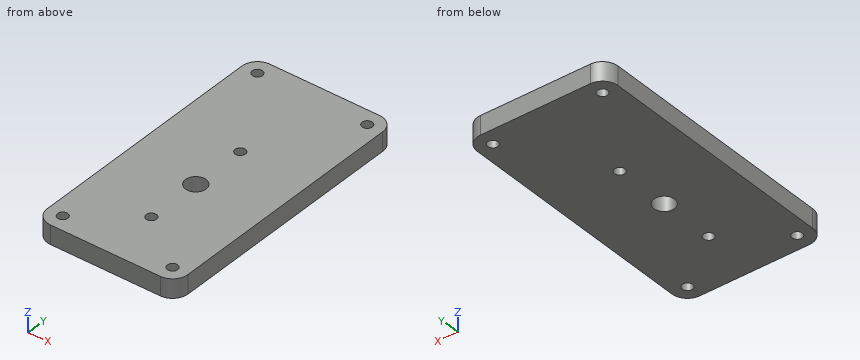
Autodesk Inventor part; units mm, degrees
ref_plane "YZ Plane" through (0, 0, 0) normal (1, 0, 0) x (0, 1, 0)
ref_plane "XZ Plane" through (0, 0, 0) normal (0, 1, 0) x (-1, 0, 0)
ref_plane "XY Plane" through (0, 0, 0) normal (0, 0, 1) x (1, 0, 0)
sketch "スケッチ1" plane through (0, 0, 0) normal (0, 0, 1) x (1, 0, 0)
  line L0 (0, 0) -> (41, 0)
  line L1 (41, 0) -> (41, -80)
  line L2 (41, -80) -> (0, -80)
  line L3 (0, -80) -> (0, 0)
  dimension "d0" = 41
  dimension "d13" = 80
extrude "押し出し1" add sketch "スケッチ1" along normal blind 5.5
sketch "スケッチ2" plane through (0, 0, 5.5) normal (0, 0, 1) x (1, 0, 0)
  line L0 (4.5, -75.5) -> (36.5, -75.5)
  line L1 (36.5, -75.5) -> (36.5, -4.5)
  line L2 (36.5, -4.5) -> (4.5, -4.5)
  line L3 (4.5, -4.5) -> (4.5, -75.5)
  line L4 (0, -80) -> (41, -80)
  line L5 (0, 0) -> (0, -80)
  dimension "d3" = 4.5
  dimension "d4" = 32
  dimension "d5" = 4.5
  dimension "d14" = 71
hole "穴1" at (4.5, -4.5, 5.5) at (36.5, -4.5, 5.5) at (36.5, -75.5, 5.5) at (4.5, -75.5, 5.5) direction (0, 0, -1) diameter 3 end through all
fillet "フィレット1" radius 4.5 4 edges at (0, 0, 2.75) (41, 0, 2.75) (0, -80, 2.75) (41, -80, 2.75)
sketch "スケッチ3" plane through (0, 0, 5.5) normal (0, 0, 1) x (1, 0, 0)
  line L0 (36.5, 0) -> (4.5, 0)
  line L1 (41, -75.5) -> (41, -4.5)
  line L2 (0, -4.5) -> (0, -75.5)
  point P0 (0, 0)
  point P1 (20.5, -47)
  dimension "d16" = 47
  dimension "d17" = 41
  dimension "d18" = 20.5
hole "穴2" at (20.5, -47, 5.5) direction (0, 0, -1) diameter 6 end through all
sketch "スケッチ4" plane through (0, 0, 5.5) normal (0, 0, 1) x (1, 0, 0)
  circle A0 centre (20.5, -47) radius 3
  point P0 (0, 0)
  point P1 (20.5, -30.785)
  point P2 (20.5, -63.215)
  dimension "d26" = 32.43
  dimension "d27" = 16.215
  dimension "d28" = 0
  dimension "d29" = 0
hole "穴3" at (20.5, -30.785, 5.5) at (20.5, -63.215, 5.5) direction (0, 0, -1) diameter 3 end through all
properties part number "上下直動t5.5_エンコーダ軸受け_CPY" material "木材 (カエデ材)"
Read the model definition and answer for the solid it produces. Units are mm, in the model's axes. Round coordinates to 2 decimals unless told otherwise and drop trailing zeros. Write each loop counter-clockwise with the first axis right and the second up, starting at its lowest first coordinate (ties: lowest second). Pieces come first, ordered by that corner, then holes. Notation, with made-up numbers: M -1,73 L 32,73 A17 ccw 32,87 Z; hole C 16,-25.5 d6. An arc over 180 degrees is marked long. Use a Markdown table: item, result.
1) The part is cut by section A-A (y = -47). Write down the section's boundary in (x, z).
Answers follow:
| item | result |
|---|---|
| outline | M 0,0 L 17.5,0 L 17.5,5.5 L 0,5.5 Z; M 23.5,0 L 41,0 L 41,5.5 L 23.5,5.5 Z |
2) Flat-ended cylindrical pins translate along their axes: pin 1 (3.5 mm diameter, centred on x = 36.5, y = -4.5, fed in from +Z); pin 2 (5 mm diameter, centred on x = 20.5, y = -47, fed in from -Z). Find the tip coordinate at first contact, or state that the pin passes through.
Answers follow:
| item | result |
|---|---|
| pin 1 | stops at z = 5.5 |
| pin 2 | passes through |
3) The part is cut by section B-B (z = 3.3). Write down the section's boundary in (x, y) (3 decimals), plus the area to 3 significant figures.
Answers follow:
| item | result |
|---|---|
| outline | M 0,-75.5 A4.5 ccw 4.5,-80 L 36.5,-80 A4.5 ccw 41,-75.5 L 41,-4.5 A4.5 ccw 36.5,0 L 4.5,0 A4.5 ccw 0,-4.5 Z; hole C 4.5,-75.5 d3; hole C 4.5,-4.5 d3; hole C 20.5,-47 d6; hole C 20.5,-63.215 d3; hole C 20.5,-30.785 d3; hole C 36.5,-75.5 d3; hole C 36.5,-4.5 d3 |
| area | 3,190 mm2 |
4) Straight lines are drawn through the part: line 1 along Y through (x, z) = (20.5, 2) (3 decimals); line 2 along Y through (x, z) = (36.5, 3); line 3 along X through (y, z) = (-75.5, 2.65). For each, find the intervals that lie inside material, in ascending order. Write a range as [from, to].
Answers follow:
| item | result |
|---|---|
| line 1 | y = [-80, -64.715], [-61.715, -50], [-44, -32.285], [-29.285, 0] |
| line 2 | y = [-80, -77], [-74, -6], [-3, 0] |
| line 3 | x = [0, 3], [6, 35], [38, 41] |
